from build123d import *

# Parameters (mm, degrees)
F0_R     = 1.85
F1_DEPTH = 0.95
F2_W     = 4.5
F2_H     = 4.2
F3_DEPTH = 3.25
F4_R     = 2.09999
F5_R     = 1.15
F6_DEPTH = 25


# Not quite as in the source:
# - a fillet or chamfer is up to 0.001 mm smaller than in the source, because OpenCascade refuses the exact size


with BuildPart() as f1:
    # F0 (on Top) → F1 (new body)
    with BuildSketch(Plane.XY):
        with BuildLine():
            Line((8.2, 1.15), (12.7, 1.15))
            Line((12.7, 1.15), (12.7, 5.35))
            Line((12.7, 5.35), (8.2, 5.35))
            Line((8.2, 5.35), (7.7320977576, 5.35))
            ThreePointArc((7.7320977576, 5.35), (7.2069912058, 5.3927015871), (6.6956833513, 5.5196842405))
            Line((6.6956833513, 5.5196842405), (4.2864144063, 6.3303157595))
            ThreePointArc((4.2864144063, 6.3303157595), (3.7751065518, 6.4572984129), (3.25, 6.5))
            ThreePointArc((3.25, 6.5), (0.9519029611, 5.5480970389), (0, 3.25))
            ThreePointArc((0, 3.25), (0.9519029611, 0.9519029611), (3.25, 0))
            ThreePointArc((3.25, 0), (3.7751065518, 0.0427015871), (4.2864144063, 0.1696842405))
            Line((4.2864144063, 0.1696842405), (6.6956833513, 0.9803157595))
            ThreePointArc((6.6956833513, 0.9803157595), (7.2069912058, 1.1072984129), (7.7320977576, 1.15))
            Line((7.7320977576, 1.15), (8.2, 1.15))
        make_face()
        with Locations((3.25, 3.25)):
            Circle(F0_R, mode=Mode.SUBTRACT)
    extrude(amount=F1_DEPTH)

    # F2 (on face) → F3 (join)
    with BuildSketch(Plane.XY.offset(0.95)):
        with Locations((10.45, 3.25)):
            Rectangle(F2_W, F2_H)
    extrude(amount=F3_DEPTH)

    # F4 (radius 2.1 in the source; OpenCascade refuses exactly that, so slightly less here)
    f4_edges = [f1.edges().sort_by_distance(p)[0] for p in [
        (10.45, 5.35, 4.2),
        (10.45, 1.15, 4.2),
    ]]
    fillet(f4_edges, radius=F4_R)

    # F5 (on face) → F6 (cut)
    with BuildSketch(Plane.YZ.offset(12.7)):
        with Locations((3.25, 2.1)):
            Circle(F5_R)
    extrude(amount=-F6_DEPTH, mode=Mode.SUBTRACT)


solid = f1.part
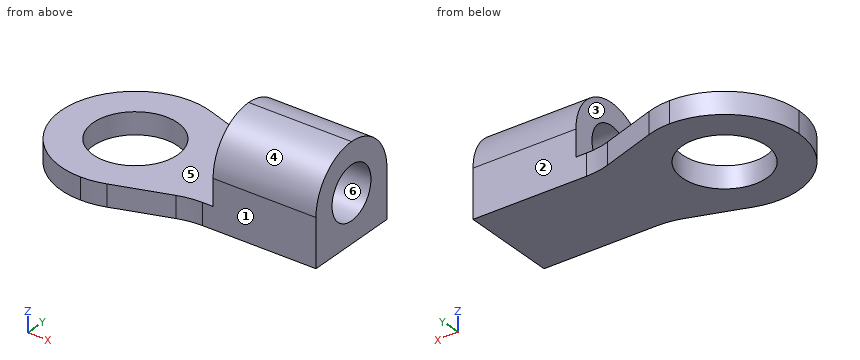
Read the model definition and answer for the solid it produces. Units are mm, in the model's axes. Face numbers are marked on the shaded views. A direction names the side the tool comes from. Give positions to 0.01 mm unless a question says otherwise; leave off trailing zeros. Write each loop counter-clockwise with the first axis right and the second up, starting at its lowest first coordinate (ties: lowest second). Pieces come first, ordered by that corner, then holes. Notation, with made-up numbers: (89.5, 66) -> (130.5, 66) arc R27 cw to (130.5, 93) -> close; hole circle Ø1 at (50, 41.5). An arc over 180 degrees is marked (long way). Answer as a JSON object with one key per item and string values. Group by question number.
1) Find section D-D (x = 2). Write down the section's boundary in (y, z), and give its area (3 significant figures).
2) Find section A-A (z = 0.65). Write down the section's boundary in (x, y).
3) Each of these flat-tipped pins is pushed along its axis until it touches: P1, Ø0.6, axis at x = 9.5, z = 1, coming from the -Y side; P2, Ø1, axis at y = 4, z = 2, coming from the -X side; P3, Ø0.6, axis at x = 9, z = 0.5, coming from the +Y side. Where does it stop, or does it pass through?
4) Consider L1, parallel to Y at x = 10.15, z = 2.1; L2, parallel to Y at x = 3.25, z = 0.35; L3, parallel to X at y = 3.25, z = 0.3. Determine where each line is inside the solid, lowest interval first. Write a range as from..to.
5) The mould has two halves that part along Y. Classify the marked faces 4, 5 and 6: +Y half, -Y half, draft (parallel to the pull), parting line (faces both ways), or undercut.
6) A tool of negligible diameter and unlimited length cuts with its end or side. For the marked faces 1, 2 and 3, from which of +Z, -Z, +X, -X, +Y, -Y can it reach the whole face along a straight path? Write none if from no direction.
7) Find section C-C (z = 1.6). Write down the section's boundary in (x, y).
Values follow:
{
 "1": {"outline": "(0.25, 0) -> (1.89, 0) -> (1.89, 0.95) -> (0.25, 0.95) -> close; (4.61, 0) -> (6.25, 0) -> (6.25, 0.95) -> (4.61, 0.95) -> close", "area": "3.11 mm2"},
 "2": {"outline": "(4.29, 0.17) -> (6.7, 0.98) arc R3.25 cw to (7.73, 1.15) -> (12.7, 1.15) -> (12.7, 5.35) -> (7.73, 5.35) arc R3.25 cw to (6.7, 5.52) -> (4.29, 6.33) arc R3.25 ccw (long way) to start; hole circle Ø3.7 at (3.25, 3.25)"},
 "3": {"P1": "stops at y = 1.15", "P2": "stops at x = 8.2", "P3": "stops at y = 5.35"},
 "4": {"L1": "y = 1.15..2.1, 4.4..5.35", "L2": "y = 0..1.4, 5.1..6.5", "L3": "x = 0..1.4, 5.1..12.7"},
 "5": {"face 4": "-Y half", "face 5": "draft", "face 6": "undercut"},
 "6": {"face 1": "+Z, -Z, +X, -Y", "face 2": "+Z, -Z, +X, +Y", "face 3": "+Z, -X, +Y, -Y"},
 "7": {"outline": "(8.2, 1.15) -> (12.7, 1.15) -> (12.7, 2.21) -> (8.2, 2.21) -> close; (8.2, 4.29) -> (12.7, 4.29) -> (12.7, 5.35) -> (8.2, 5.35) -> close"}
}
